Geometry check sheet. Reference: the model listing, model coordinates, mm. A direction names the side the tool comes from. Give positions to 0.01 mm unless a question says otherwise; leave off trailing zeros. Loops run counter-clockwise (first coordinate to the right, second up) from the corner with the lowest first, then second, coordinate; pieces in that order, holes last.
```python
from build123d import *

# Parameters (mm, degrees)
SKETCH_1_R          = 30
EXTRUDE_1_DEPTH     = 20
EXTRUDE_2_DEPTH     = 10
EXTRUDE_3_DEPTH     = 10
CUT_EXTRUDE_1_DEPTH = 10
SKETCH_5_R          = 1.45
CUT_EXTRUDE_2_DEPTH = 3
SKETCH_7_R          = 3.5
CUT_EXTRUDE_4_DEPTH = 47.904157598
SKETCH_8_R          = 5
CUT_EXTRUDE_5_DEPTH = 3


with BuildPart() as part:
    # Sketch 1 → Extrude 1 (new body)
    with BuildSketch(Plane.XY):
        Circle(SKETCH_1_R)
    extrude(amount=EXTRUDE_1_DEPTH)

    # Sketch 2 → Extrude 2 (add)
    with BuildSketch(Plane(origin=(0, 0, 0), x_dir=(-1, 0, 0), z_dir=(0, 0, -1))):
        with BuildLine():
            Line((12.5, 30), (0, 30))
            ThreePointArc((0, 30), (6.397131834, 29.310010309), (12.5, 27.271780287))
            Line((12.5, 27.271780287), (12.5, 30))
        make_face()
        with BuildLine():
            Line((0, 30), (-12.5, 30))
            Line((-12.5, 30), (-12.5, 27.271780287))
            ThreePointArc((-12.5, 27.271780287), (-6.397131834, 29.310010309), (0, 30))
        make_face()
    extrude(amount=-EXTRUDE_2_DEPTH)

    # Sketch 3 → Extrude 3 (add)
    with BuildSketch(Plane.XY.offset(10)):
        with BuildLine():
            Line((-12.5, 30), (-12.5, 27.271780287))
            ThreePointArc((-12.5, 27.271780287), (-6.397131834, 29.310010309), (0, 30))
            Line((0, 30), (-12.5, 30))
        make_face()
        with BuildLine():
            ThreePointArc((0, 30), (6.397131834, 29.310010309), (12.5, 27.271780287))
            Line((12.5, 27.271780287), (12.5, 30))
            Line((12.5, 30), (0, 30))
        make_face()
    extrude(amount=EXTRUDE_3_DEPTH)

    # Sketch 4 → Cut-Extrude 1 (cut)
    with BuildSketch(Plane(origin=(0, 0, 0), x_dir=(-1, 0, 0), z_dir=(0, 0, -1))):
        with BuildLine():
            Line((-12.5, 30), (-12.5, 27.271780287))
            ThreePointArc((-12.5, 27.271780287), (-6.397131834, 29.310010309), (0, 30))
            Line((0, 30), (-12.5, 30))
        make_face()
        with BuildLine():
            ThreePointArc((0, 30), (6.397131834, 29.310010309), (12.5, 27.271780287))
            Line((12.5, 27.271780287), (12.5, 30))
            Line((12.5, 30), (0, 30))
        make_face()
    extrude(amount=-CUT_EXTRUDE_1_DEPTH, mode=Mode.SUBTRACT)

    # Sketch 5 → Cut-Extrude 2 (cut)
    with BuildSketch(Plane(origin=(0, 30, 0), x_dir=(1, 0, 0), z_dir=(0, 1, 0))):
        with Locations(Location((-3.75, -16.5, 0), (0, 0, 270))):
            Circle(SKETCH_5_R)
        with Locations(Location((3.75, -16.5, 0), (0, 0, 270))):
            Circle(SKETCH_5_R)
    extrude(amount=-CUT_EXTRUDE_2_DEPTH, mode=Mode.SUBTRACT)

    # Sketch 7 → Cut-Extrude 4 (cut, through all)
    with BuildSketch(Plane.XY.offset(20)):
        Circle(SKETCH_7_R)
    extrude(amount=-CUT_EXTRUDE_4_DEPTH, mode=Mode.SUBTRACT)

    # Sketch 8 → Cut-Extrude 5 (cut)
    with BuildSketch(Plane.XY.offset(20)):
        Circle(SKETCH_8_R)
    extrude(amount=-CUT_EXTRUDE_5_DEPTH, mode=Mode.SUBTRACT)


solid = part.part
```
1) Sectioned sample at D-D on y = 11. Enter the section's corners in (x, z), plus the area to 3 significant figures.
2) Mould release check, pull along X, two halves, no side actions. Record for faces 5 (the flat face through (4, 27, 16)), 6 (the flat face through (-9, 29, 10)), 7 (the flat face through (-12.5, 29, 15)), 8 (the flat face through (12.5, 29, 15)): +X half, -X half, draft (parallel to the pull), parting line (faces both ways), or undercut.
3) Sectioned sample at C-C on z = 6.25. Enter the section's corners in (x, y).
4) Depth check by flat-ended pin: P1, Ø1, axis at x = 4, z = 2.5, coming from the -Y side; P2, Ø2.5, axis at x = 3.75, z = 16.5, coming from the +Y side; P3, Ø1.4, axis at y = 28, z = 13, coming from the -X side; P4, Ø3, axis at x = -1, y = -1, coming from the +Z side. Enter the tip coordinate at first touch or a pass-through.
5) Sectioned sample at A-A on y = 0. Enter the section's corners in (x, z).
6) Scan lines: line 1 along X through (y, z) = (28, 16.5); line 2 along Y through (x, z) = (0, 11.75); line 3 along Y through (x, z) = (0, 19.4). Record each from-to range of solid material in increasing order.
7) Tool access check on faces 1 (the flat face through (10, 29, 10)), 2 (the flat face through (2.2, -3.3, 17)), 3 (the flat face through (0, 30, 15)), 4 (the cylindrical face through (4.19, 28.52, 17.88)). Record the directions out of +Z, -Z, +X, -X, +Y, -Y that give a thin tool (end or side, any length) a straight path to the whole face; none if there is none.
Determined:
1. outline: (-27.91, 0) - (27.91, 0) - (27.91, 20) - (-27.91, 20) - close
1. area: 1,120 mm2
2. face 5: undercut
2. face 6: draft
2. face 7: -X half
2. face 8: +X half
3. outline: circle Ø60 at (0, 0); hole circle Ø7 at (0, 0)
4. P1: stops at y = -29.8
4. P2: stops at y = 27
4. P3: stops at x = -12.5
4. P4: passes through
5. outline: (-30, 0) - (-3.5, 0) - (-3.5, 17) - (-5, 17) - (-5, 20) - (-30, 20) - close; (3.5, 0) - (30, 0) - (30, 20) - (5, 20) - (5, 17) - (3.5, 17) - close
6. line 1: x = -12.5 to -5.2, -2.3 to 2.3, 5.2 to 12.5
6. line 2: y = -30 to -3.5, 3.5 to 30
6. line 3: y = -30 to -5, 5 to 30
7. face 1: -Z, +X, +Y
7. face 2: +Z
7. face 3: +Z, -Z, +X, -X, +Y
7. face 4: +Y
